Verification items for the finished model (mm, model axes). Face numbers are marked on the shaded views. A direction names the side the tool comes from. Give positions to 0.01 mm unless a question says otherwise; leave off trailing zeros. Order: outer loops, then holes, each group sorted by start corner. A loop starts at its lowest first (then second) coordinate and runs counter-clockwise, first axis right, second up. Notation, with made-up numbers: M 47.25,-22.75 L 80.25,-22.75 A28 ccw 80.25,12.25 Z; hole C -6.75,45 d2. An arc over 180 degrees is marked long. Answer as a JSON object with one key per item and string values.
```python
from build123d import *

# Parameters (mm, degrees)
SKETCH_1_W      = 16
SKETCH_1_H      = 6.782608696
SKETCH_1_R      = 1.3
EXTRUDE_1_DEPTH = 2
SKETCH_2_R      = 2.8
EXTRUDE_2_DEPTH = 7.5
SKETCH_3_R      = 2.05
EXTRUDE_3_DEPTH = 4
SKETCH_4_R      = 0.65
EXTRUDE_4_DEPTH = 3


with BuildPart() as part:
    # 草图1 → 凸台-拉伸1 (new body)
    with BuildSketch(Plane(origin=(0, 0, 0), x_dir=(1, 0, 0), z_dir=(0, 1, 0))):
        Rectangle(SKETCH_1_W, SKETCH_1_H)
        with Locations(Location((-6.05, 0, 0), (0, 0, 270))):
            Circle(SKETCH_1_R, mode=Mode.SUBTRACT)
        with Locations(Location((6.05, 0, 0), (0, 0, 270))):
            Circle(SKETCH_1_R, mode=Mode.SUBTRACT)
    extrude(amount=EXTRUDE_1_DEPTH)

    # 草图2 → 凸台-拉伸2 (add)
    with BuildSketch(Plane(origin=(0, 2, 0), x_dir=(1, 0, 0), z_dir=(0, 1, 0))):
        with Locations(Location((0, 0, 0), (0, 0, 270))):
            Circle(SKETCH_2_R)
    extrude(amount=EXTRUDE_2_DEPTH)

    # 草图3 → 凸台-拉伸3 (add)
    with BuildSketch(Plane.XZ):
        with Locations(Location((0, 0, 0), (0, 0, 90))):
            Circle(SKETCH_3_R)
    extrude(amount=EXTRUDE_3_DEPTH)

    # 草图4 → 凸台-拉伸4 (add)
    with BuildSketch(Plane.XZ.offset(4)):
        with Locations(Location((0, 0, 0), (0, 0, 270))):
            Circle(SKETCH_4_R)
    extrude(amount=EXTRUDE_4_DEPTH)


solid = part.part
```
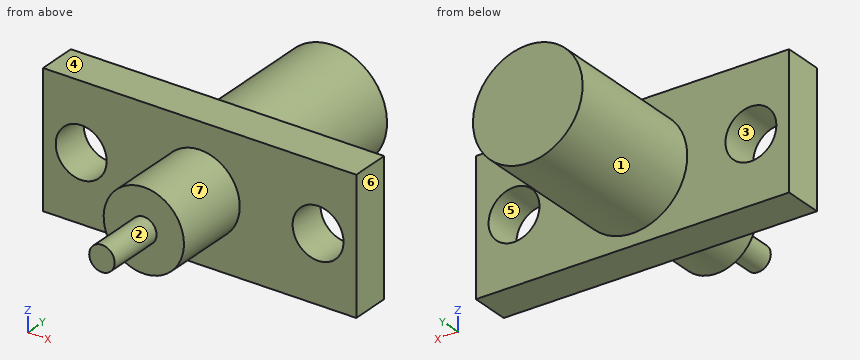
Q1. Section check B-B on x = 6.05. Record the cut outline in (y, z), then the cut area to 3 significant figures.
Resolved:
{"outline": "M 0,-3.39 L 2,-3.39 L 2,-1.3 L 0,-1.3 Z; M 0,1.3 L 2,1.3 L 2,3.39 L 0,3.39 Z", "area": "8.37 mm²"}
Q2. Gauge pin test, flat ends, axial feed: pin 1 Ø4 at (x, z) = (6.05, 0) entering from +Y; pin 2 Ø1 at (x, y) = (-1.5, -3.5) entering from -Z; pin 3 Ø1 at (y, z) = (6, -0.5) entering from -X; pin 4 Ø1.5 at (x, y) = (4, 5.5) entering from +Z. Record the tip position at first contact, or that the pin passes through.
Resolved:
{"pin 1": "stops at y = 2", "pin 2": "stops at z = -1.79", "pin 3": "stops at x = -2.8", "pin 4": "passes through"}
Q3. Release check for a two-part mould opening along Z. For the marked faces 4, 5, 6 and 7 record: +Z half, -Z half, draft (parallel to the pull), parting line (faces both ways), or undercut.
Resolved:
{"face 4": "+Z half", "face 5": "undercut", "face 6": "draft", "face 7": "parting line"}
Q4. Section check A-A on z = 0. Record the cut outline in (x, y), then the cut area to 3 significant figures.
Resolved:
{"outline": "M -8,0 L -7.35,0 L -7.35,2 L -8,2 Z; M -4.75,0 L -2.05,0 L -2.05,-4 L -0.65,-4 L -0.65,-7 L 0.65,-7 L 0.65,-4 L 2.05,-4 L 2.05,0 L 4.75,0 L 4.75,2 L 2.8,2 L 2.8,9.5 L -2.8,9.5 L -2.8,2 L -4.75,2 Z; M 7.35,0 L 8,0 L 8,2 L 7.35,2 Z", "area": "83.9 mm²"}
Q5. Section check C-C on y = 0.25. Record the cut outline in (x, z), then the cut area to 3 significant figures.
Resolved:
{"outline": "M -8,-3.39 L 8,-3.39 L 8,3.39 L -8,3.39 Z; hole C -6.05,0 d2.6; hole C 6.05,0 d2.6", "area": "97.9 mm²"}
Q6. Section check D-D on x = 0. Record the cut outline in (y, z), then the cut area to 3 significant figures.
Resolved:
{"outline": "M -7,-0.65 L -4,-0.65 L -4,-2.05 L 0,-2.05 L 0,-3.39 L 2,-3.39 L 2,-2.8 L 9.5,-2.8 L 9.5,2.8 L 2,2.8 L 2,3.39 L 0,3.39 L 0,2.05 L -4,2.05 L -4,0.65 L -7,0.65 Z", "area": "75.9 mm²"}
Q7. Material ranges on L1, parallel to Y at x = 4.5, z = -2.5; L2, parallel to X at y = 8.5, z = 0; L3, parallel to Y at x = 2, z = -1.75, recorded low to high.
Resolved:
{"L1": "y = 0 to 2", "L2": "x = -2.8 to 2.8", "L3": "y = 0 to 9.5"}
Q8. Tool access check on the marked faces 1, 2 and 3. Record the directions out of +Z, -Z, +X, -X, +Y, -Y that give a thin tool (end or side, any length) a straight path to the whole face; none if there is none.
Resolved:
{"face 1": "+Y", "face 2": "-Y", "face 3": "+Y, -Y"}
